Build history of the part. All positions in model axes, mm. Coordinates: 2 decimals unless noted, no trailing zeros. Loops run counter-clockwise (first coordinate to the right, second up) from the corner with the lowest first, then second, coordinate; pieces in that order, holes last. Notation, with made-up numbers: (19.5, 10) - (23.5, 10) arc R37 cw to (23.5, 49) - close; hole circle Ø9 at (30, 25.5). An arc over 180 degrees is marked (long way). One line per item, written item: value.
Autodesk Fusion 360 part; units mm, degrees
sketch "Sketch1" plane through (0, 0, 0) normal (0, 0, 1) x (1, 0, 0)
  line L0 (0, 0) -> (0, 230)
  line L1 (0, 230) -> (267, 230)
  line L2 (267, 230) -> (300, 210.9474)
  line L3 (300, 19.0526) -> (267, 0)
  line L4 (267, 0) -> (0, 0)
  line L5 (300, 210.9474) -> (300, 19.0526)
  dimension "d1" = 230
  dimension "d2" = 267
  dimension "d3" = 33
  dimension "d4" = 150
  dimension "d5" = 150
extrude "Extrude1" add sketch "Sketch1" along normal blind 5
sketch "Sketch2" plane through (0, 0, 5) normal (0, 0, 1) x (-1, 0, 0)
  line L0 (-300, -210.9474) -> (-267, -230)
  line L1 (-267, -230) -> (0, -230)
  line L2 (0, -230) -> (0, 0)
  line L3 (0, 0) -> (-267, 0)
  line L4 (-267, 0) -> (-300, -19.0526)
  line L5 (-300, -19.0526) -> (-300, -210.9474)
  ellipse E0 centre (-219.2825, -65.8758) end of major axis (-229.95, -65.8758) minor radius 15
  line L6 (-208.6151, -65.8758) -> (-229.95, -65.8758) construction
  line L7 (-219.2825, -50.8758) -> (-219.2825, -80.8758) construction
  dimension "d8" = 30
extrude "Extrude2" cut sketch "Sketch2" against normal through all contours E0
pattern_linear "R-Pattern1" count 3 spacing 20 along (0, 1, 0) of "Extrude2"
sketch "Sketch3" plane through (0, 0, 5) normal (0, 0, 1) x (-1, 0, 0)
  ellipse E0 centre (-219.2825, -85.8758) end of major axis (-219.2825, -100.8758) minor radius 10.6675 (-227.2336, -75.8758) -> (-227.2336, -95.8758) ccw
  ellipse E1 centre (-219.2825, -65.8758) end of major axis (-219.2825, -80.8758) minor radius 10.6675 (-211.3315, -75.8758) -> (-227.2336, -75.8758) ccw
  ellipse E2 centre (-219.2825, -85.8758) end of major axis (-219.2825, -100.8758) minor radius 10.6675 (-211.3315, -95.8758) -> (-211.3315, -75.8758) ccw
  ellipse E3 centre (-219.2825, -105.8758) end of major axis (-219.2825, -120.8758) minor radius 10.6675 (-227.2336, -95.8758) -> (-211.3315, -95.8758) ccw
  line L0 (-300, -210.9474) -> (-267, -230)
  line L1 (-267, -230) -> (0, -230)
  line L2 (0, -230) -> (0, 0)
  line L3 (0, 0) -> (-267, 0)
  line L4 (-267, 0) -> (-300, -19.0526)
  line L5 (-300, -19.0526) -> (-300, -210.9474)
  line L6 (0, -40) -> (-120, -40)
  line L7 (-120, -40) -> (-120, -30)
  line L8 (-120, -30) -> (0, -30)
  line L9 (0, -30) -> (0, -40)
  line L10 (0, -210) -> (-120, -210)
  line L11 (-120, -210) -> (-120, -200)
  line L12 (-120, -200) -> (0, -200)
  line L13 (0, -200) -> (0, -210)
  line L14 (-183, -210) -> (-190, -210)
  line L15 (-190, -210) -> (-190, -30)
  line L16 (-190, -30) -> (-183, -30)
  line L17 (-183, -30) -> (-183, -210)
  line L18 (-190, -160) -> (-183, -160)
  line L19 (-190, -80) -> (-183, -80)
  dimension "d15" = 30
  dimension "d16" = 10
  dimension "d18" = 120
  dimension "d19" = 20
  dimension "d21" = 10
  dimension "d22" = 180
  dimension "d26" = 30
  dimension "d30" = 180
  dimension "d31" = 7
  dimension "d33" = 70
  dimension "d34" = 30
  dimension "d35" = 110
  dimension "d36" = 80
  dimension "d37" = 20
  dimension "d38" = 50
extrude "Extrude4" cut sketch "Sketch3" against normal through all contours L2 L10 L11 L12 L13 | L2 L6 L7 L8 L9
extrude "Extrude6" cut sketch "Sketch3" against normal through all contours L15 L17 L18 L19
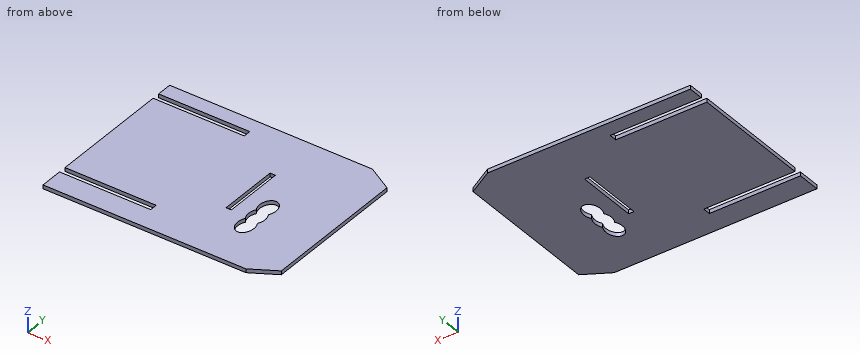
Item 1: Drop flat-ended pins along their axis: P1, Ø2.5, axis at x = 74, z = 1.5, coming from the -Y side; P2, Ø1.5, axis at y = 36, z = 1.5, coming from the -X side. Give the stop position or say it passes through.
Check result:
P1: stops at y = 0
P2: stops at x = 120
Item 2: Cut at A-A, the plane x = 84.5. Write the cut outline in (y, z), then the cut area to 3 significant figures.
Check result:
outline: (0, 0) - (30, 0) - (30, 5) - (0, 5) - close; (40, 0) - (200, 0) - (200, 5) - (40, 5) - close; (210, 0) - (230, 0) - (230, 5) - (210, 5) - close
area: 1,050 mm^2
Item 3: Cut at B-B, the plane z = 4.15. Give the number of separate pieces and of enclosed holes in the cut face, then the cut area to 3 significant figures.
Check result:
separate pieces: 1
enclosed holes: 2
area: 64,100 mm^2
Item 4: Probe probe 1 along Y at (x, z) = (56, 4.65); probe 2 along X at (y, z) = (128, 3.2); probe 3 along X at (y, z) = (112.5, 0.85). List the from-to ranges inside material, lowest first. Write a range as from..to.
Check result:
probe 1: y = 0..30, 40..200, 210..230
probe 2: x = 0..183, 190..300
probe 3: x = 0..183, 190..209.71, 228.85..300
